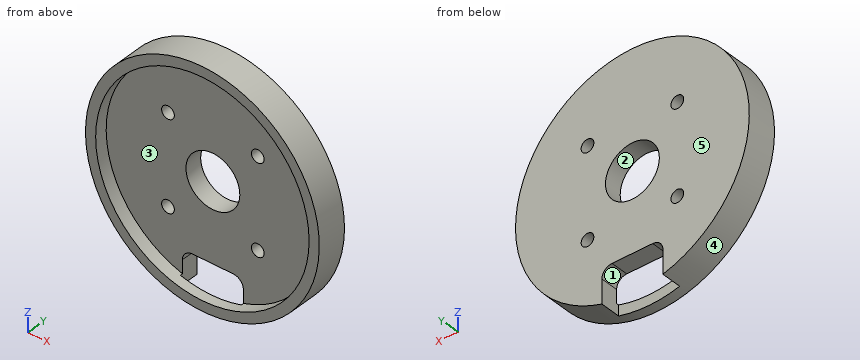
```python
from build123d import *

# Parameters (mm, degrees)
SKETCH_1_R          = 23
EXTRUDE_1_DEPTH     = 6
SKETCH_2_R          = 21
SKETCH_2_R_2        = 5.3
CUT_EXTRUDE_1_DEPTH = 2.5
SKETCH_2_3_R        = 5.3
CUT_EXTRUDE_2_DEPTH = 34.075670817
CUT_EXTRUDE_START   = -4
CUT_EXTRUDE_3_DEPTH = 4
M3X0_51_D           = 2.5


with BuildPart() as part:
    # Sketch 1 → Extrude 1 (new body)
    with BuildSketch(Plane(origin=(0, 0, 0), x_dir=(1, 0, 0), z_dir=(0, 1, 0))):
        with Locations(Location((0, 0, 0), (0, 0, 270))):
            Circle(SKETCH_1_R)
    extrude(amount=EXTRUDE_1_DEPTH)

    # Sketch 2 → Cut-Extrude 1 (cut)
    # profile 1 of 2: a face of its own
    with BuildSketch(Plane.XZ):
        with Locations(Location((0, 0, 0), (0, 0, 270))):
            Circle(SKETCH_2_R)
        Circle(SKETCH_2_R_2, mode=Mode.SUBTRACT)
    # profile 2 of 2: a face of its own
    with BuildSketch(Plane.XZ):
        Circle(SKETCH_2_R_2)
    extrude(amount=-CUT_EXTRUDE_1_DEPTH, mode=Mode.SUBTRACT)

    # Sketch 2_3 → Cut-Extrude 2 (cut, through all)
    with BuildSketch(Plane.XZ):
        with Locations(Location((0, 0, 0), (0, 0, 270))):
            Circle(SKETCH_2_3_R)
    extrude(amount=-CUT_EXTRUDE_2_DEPTH, mode=Mode.SUBTRACT)

    # Sketch 4 → Cut-Extrude 3 (cut)
    with BuildSketch(Plane(origin=(0, 6, 0), x_dir=(1, 0, 0), z_dir=(0, 1, 0)).offset(CUT_EXTRUDE_START)):
        with BuildLine():
            Line((-6, 22.203603311), (-6, 17.5))
            ThreePointArc((-6, 17.5), (-5.414213562, 16.085786438), (-4, 15.5))
            Line((-4, 15.5), (4, 15.5))
            ThreePointArc((4, 15.5), (5.414213562, 16.085786438), (6, 17.5))
            Line((6, 17.5), (6, 22.203603311))
            ThreePointArc((6, 22.203603311), (0, 23), (-6, 22.203603311))
        make_face()
    extrude(amount=CUT_EXTRUDE_3_DEPTH, mode=Mode.SUBTRACT)

    # M3x0.51 (through all)
    with Locations(Plane(origin=(0, 6, 0), x_dir=(1, 0, 0), z_dir=(0, 1, 0))):
        with Locations((-8.838834765, 8.838834765), (8.838834765, 8.838834765), (8.838834765, -8.838834765), (-8.838834765, -8.838834765)):
            Hole(M3X0_51_D / 2)


solid = part.part
```
Build history of the part. All positions in model axes, mm. Face numbers are marked on the shaded views. A direction names the side the tool comes from. Coordinates: 2 decimals unless noted, no trailing zeros. Order: outer loops, then holes, each group sorted by start corner. A loop starts at its lowest first (then second) coordinate and runs counter-clockwise, first axis right, second up. Notation, with made-up numbers: M -3,57.5 L 10,57.5 A36 cw 10,94.5 Z; hole C 76.25,-32.75 d5. An arc over 180 degrees is marked long. One line per question, with ' | ' between items. Start each with the question number.
1. Mould opens along Z. For the marked faces 3, 4 and 5 say: +Z half, -Z half, draft (parallel to the pull), parting line (faces both ways), or undercut.
2. Wall check: line 1 along X through (y, z) = (4.8, 0); line 2 along X through (y, z) = (5, 9); line 3 along X through (y, z) = (2.65, 9.5). Give the ranges that are in metal, low to high. Write a range as [from, to].
3. Cut at D-D (z = -12.5). Write the cut outline in (x, y), plus the area to 3 significant figures.
4. Cut at A-A (x = 0). Write the cut outline in (y, z), plus the area to 3 significant figures.
5. Cut at C-C (y = 3.9). Write the cut outline in (x, z), plus the area to 3 significant figures.
6. Tool access for the marked faces 1 and 2: list every direction of +Z, -Z, +X, -X, +Y, -Y with a clear straight run to the whole face (end or side of a thin tool).
7. Cut at B-B (z = 0). Write the cut outline in (x, y).
8. Flat gauge pins, fed straight in: P1, Ø2, axis at y = 3.5, z = 3, coming from the -X side; P2, Ø3, axis at x = -8.84, z = 8.84, coming from the -Y side; P3, Ø2, axis at y = 1.5, z = -0.5, coming from the +X side. Where does each tip first touch, or does it go through?
The answers:
1) face 3: undercut | face 4: parting line | face 5: draft
2) line 1: x = [-23, -5.3], [5.3, 23] | line 2: x = [-21.17, -10.08], [-7.6, 7.6], [10.08, 21.17] | line 3: x = [-20.95, -9.9], [-7.78, 7.78], [9.9, 20.95]
3) outline: M -19.31,0 L -16.87,0 L -16.87,2.5 L 16.87,2.5 L 16.87,0 L 19.31,0 L 19.31,6 L -19.31,6 Z | area: 147 mm2
4) outline: M 0,-23 L 2,-23 L 2,-21 L 0,-21 Z; M 0,21 L 2.5,21 L 2.5,5.3 L 6,5.3 L 6,23 L 0,23 Z; M 2.5,-15.5 L 6,-15.5 L 6,-5.3 L 2.5,-5.3 Z | area: 107 mm2
5) outline: M -6,-22.2 L -6,-17.5 A2 cw -4,-15.5 L 4,-15.5 A2 cw 6,-17.5 L 6,-22.2 A23 ccw long Z; hole C -8.84,-8.84 d2.5; hole C -8.84,8.84 d2.5; hole C 0,0 d10.6; hole C 8.84,-8.84 d2.5; hole C 8.84,8.84 d2.5 | area: 1,470 mm2
6) face 1: -Z, +Y, -Y | face 2: +Y, -Y
7) outline: M -23,0 L -21,0 L -21,2.5 L -5.3,2.5 L -5.3,6 L -23,6 Z; M 5.3,2.5 L 21,2.5 L 21,0 L 23,0 L 23,6 L 5.3,6 Z
8) P1: stops at x = -22.91 | P2: stops at y = 2.5 | P3: stops at x = 23
